```python
from build123d import *

# Parameters (mm, degrees)
SKETCH1_W           = 129
SKETCH1_H           = 74
BOSS_EXTRUDE1_DEPTH = 2
SKETCH2_R           = 3.5
CUT_EXTRUDE1_DEPTH  = 3


with BuildPart() as part:
    # Sketch1 → Boss-Extrude1 (new body)
    with BuildSketch(Plane(origin=(0, 0, 0), x_dir=(1, 0, 0), z_dir=(0, 1, 0))):
        with Locations((64.5, -37)):
            Rectangle(SKETCH1_W, SKETCH1_H)
    extrude(amount=BOSS_EXTRUDE1_DEPTH)

    # Sketch2 → Cut-Extrude1 (cut, through all)
    with BuildSketch(Plane.XZ):
        with Locations((79, 21)):
            Circle(SKETCH2_R)
        with Locations((79, 53)):
            Circle(SKETCH2_R)
    extrude(amount=-CUT_EXTRUDE1_DEPTH, mode=Mode.SUBTRACT)


solid = part.part
```
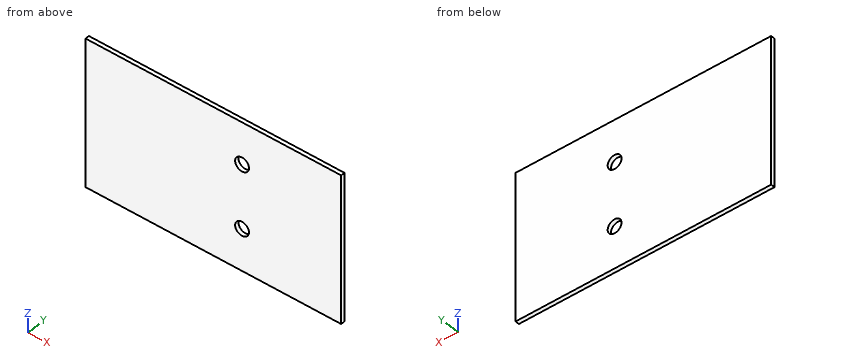
Verification items for the finished model (mm, model axes). Coordinates: 2 decimals unless noted, no trailing zeros. Loops run counter-clockwise (first coordinate to the right, second up) from the corner with the lowest first, then second, coordinate; pieces in that order, holes last. Notation, with made-up numbers: (11, 82) -> (67, 82) arc R32 ccw to (67, 113) -> close; hole circle Ø3 at (36.5, 2.5). An arc over 180 degrees is marked (long way). Answer in a Markdown table with one row per item. Add a question column.
1. Section check B-B, the plane z = 53. Enter the section's corners in (x, y).
2. Depth check by flat-ended pin: P1, Ø6.5, axis at x = 79, z = 53, coming from the -Y side. Enter the tip coordinate at first touch or a pass-through.
3. Material ranges on probe 1 along Z at (x, y) = (79, 0.5), recorded low to high. Write a range as [from, to].
4. Section check A-A, the plane x = 79. Enter the section's corners in (y, z), then the cut area to 3 significant figures.
Derived:
| question | item | result |
|---|---|---|
| 1 | outline | (0, 0) -> (75.5, 0) -> (75.5, 2) -> (0, 2) -> close; (82.5, 0) -> (129, 0) -> (129, 2) -> (82.5, 2) -> close |
| 2 | P1 | passes through |
| 3 | probe 1 | z = [0, 17.5], [24.5, 49.5], [56.5, 74] |
| 4 | outline | (0, 0) -> (2, 0) -> (2, 17.5) -> (0, 17.5) -> close; (0, 24.5) -> (2, 24.5) -> (2, 49.5) -> (0, 49.5) -> close; (0, 56.5) -> (2, 56.5) -> (2, 74) -> (0, 74) -> close |
| 4 | area | 120 mm² |
